Design review of the part built by this model. Coordinates are the model's own, in mm. A direction names the side the tool comes from. Coordinates: 2 decimals unless noted, no trailing zeros. Write each loop counter-clockwise with the first axis right and the second up, starting at its lowest first coordinate (ties: lowest second). Pieces come first, ordered by that corner, then holes. Notation, with made-up numbers: (-12, 73) - (18, 73) arc R9 cw to (18, 77) - close; hole circle Ø11 at (-23.5, -24). An arc over 180 degrees is marked (long way). One line per item, written item: value.
from build123d import *

# Parameters (mm, degrees)
F0_W     = 25.4
F0_H     = 7.9375
F3_DEPTH = 11.90625
F6_DEPTH = 17.4625


with BuildPart() as f1:
    # F0 (on Front) → F1 (revolve)
    with BuildSketch(Plane.XZ):
        with Locations((12.7, 3.96875)):
            Rectangle(F0_W, F0_H)
    revolve(axis=Axis((12.7, 0, 0), (1, 0, 0)))

    # F2 (on Right) → F3 (join)
    with BuildSketch(Plane.YZ):
        Polygon((6.874077, 11.90625), (-6.874077, 11.90625), (-13.748153, 0), (-6.874077, -11.90625), (6.874077, -11.90625), (13.748153, 0), align=None)
    extrude(amount=F3_DEPTH)

    # F5 (on offset) → F6 (join)
    with BuildSketch(Plane.YZ.offset(24.60625)):
        Polygon((6.874077, -11.90625), (13.748153, 0), (6.874077, 11.90625), (-6.874077, 11.90625), (-13.748153, 0), (-6.874077, -11.90625), align=None)
    extrude(amount=F6_DEPTH)

    # F7 (on Front) → F8 (revolve, cut)
    with BuildSketch(Plane.XZ):
        Polygon((0, 18.750624), (0, 11.90625), (3.951601, 18.750624), align=None)
        Polygon((7.954649, 18.750624), (11.90625, 11.90625), (11.90625, 18.750624), align=None)
        Polygon((24.60625, 18.750624), (24.60625, 11.90625), (28.557851, 18.750624), align=None)
        Polygon((42.06875, 11.90625), (42.06875, 18.750624), (38.117149, 18.750624), align=None)
    revolve(axis=Axis((39.392542, 0, 0), (1, 0, 0)), mode=Mode.SUBTRACT)


solid = f1.part
1. Mouldability with a two-part tool opening along X and no side actions: class faces 1 (the face through (11.65, 6.2, 10.68)), 2 (the face through (0.258, -12.354, 0.03)), 3 (the face through (5.87, -10.36, -5.87)) as released by +X, released by -X, zero draft, split by the parting line, or undercut.
Answer block:
face 1: undercut
face 2: released by -X
face 3: zero draft
2. Consider section A-A, the plane x = 28.5. Write out the cut boundary in (y, z), then the cut area to 3 significant figures.
Answer block:
outline: (-13.75, 0) - (-6.87, -11.91) - (6.87, -11.91) - (13.75, 0) - (6.87, 11.91) - (-6.87, 11.91) - close
area: 491 mm^2
3. For faces 4 (the face through (24.865, -6.151, 10.714)), 5 (the face through (0.258, 6.203, 10.684)), 6 (the face through (24.606, 2, -8)), 7 (the face through (11.65, -12.35, 0.03)), list the 3-axis set-ups (+Z, -Z, +X, -X, +Y, -Y) from which the entire face can be reached by the end or side of a thin tool; tool diameter is ignored.
Answer block:
face 4: +Z, -Y
face 5: +Z, -X, +Y
face 6: none
face 7: -Y
4. Insertion check: pin 1 Ø6 at (x, y) = (13, -10) entering from +Z; pin 2 Ø4 at (x, z) = (28, 8.5) entering from -Y. Each pin has a flat end and moves straight along its axis. Give the tip position at first contact, or say it passes through.
Answer block:
pin 1: stops at z = 10.67
pin 2: stops at y = -10
5. Wall thickness on line 1 along X through (y, z) = (-0.5, -8); line 2 along X through (y, z) = (12, 2.25); line 3 along Y through (x, z) = (13.5, 2): over which ranges is each line inside the solid? List them lowest first.
Answer block:
line 1: x = 0 to 11.91, 24.61 to 42.07
line 2: x = 0.17 to 11.73, 24.78 to 41.89
line 3: y = -7.68 to 7.68
